Design review of the part built by this model. Coordinates are the model's own, in mm. A direction names the side the tool comes from. Coordinates: 2 decimals unless noted, no trailing zeros. Order: outer loops, then holes, each group sorted by start corner. A loop starts at its lowest first (then second) coordinate and runs counter-clockwise, first axis right, second up. Notation, with made-up numbers: M -3.5,52 L 50.5,52 A20 ccw 50.5,78 Z; hole C 28,-39 d9. An arc over 180 degrees is marked long. Use CSV: the item, a comma, the result in double quotes.
```python
from build123d import *

# Parameters (mm, degrees)
CROQUIS1_W                = 209.55
CROQUIS1_H                = 146.05
SALIENTE_EXTRUIR1_DEPTH   = 3.1242
CROQUIS2_R                = 1.3335
CORTAR_EXTRUIR1_DEPTH     = 128.750584639
CROQUIS9_R                = 1.27
CORTAR_EXTRUIR6_DEPTH     = 128.750584639
CORTAR_EXTRUIR2_DEPTH     = 128.750584639
CROQUIS5_R                = 1.651
DRIVER_DEPTH              = 128.750584639
CROQUIS6_R                = 1.651
RASPI_DEPTH               = 128.750584639
CROQUIS8_R                = 1.27
DIFERENCIAL_TRASERO_DEPTH = 128.750584639
CROQUIS7_R                = 1.5875
CROQUIS7_W                = 11.1125
CROQUIS7_H                = 2.9972
CORTAR_EXTRUIR7_DEPTH     = 128.750584639
CROQUIS10_R               = 1.651
CROQUIS10_W               = 22.606
CROQUIS10_H               = 11.9888
CORTAR_EXTRUIR10_DEPTH    = 128.750584639
CORTAR_EXTRUIR11_DEPTH    = 128.750584639


with BuildPart() as part:
    # Croquis1 → Saliente-Extruir1 (new body)
    with BuildSketch(Plane.XY):
        Rectangle(CROQUIS1_W, CROQUIS1_H)
    extrude(amount=SALIENTE_EXTRUIR1_DEPTH)

    # Croquis2 → Cortar-Extruir1 (cut, through all)
    with BuildSketch(Plane.XY.offset(3.1242)):
        with BuildLine():
            ThreePointArc((80.5799125, 60.7314), (79.928852882, 61.877042778), (78.6114125, 61.904002767))
            Line((78.6114125, 61.904002767), (78.6114125, 59.558797233))
            ThreePointArc((78.6114125, 59.558797233), (79.928852882, 59.585757222), (80.5799125, 60.7314))
        make_face()
        with BuildLine():
            Line((78.6114125, 59.558797233), (78.6114125, 61.904002767))
            ThreePointArc((78.6114125, 61.904002767), (77.9129125, 60.7314), (78.6114125, 59.558797233))
        make_face()
        with Locations(Location((79.2464125, -60.7314, 0), (0, 0, 180))):
            Circle(CROQUIS2_R)
    extrude(amount=-CORTAR_EXTRUIR1_DEPTH, mode=Mode.SUBTRACT)

    # Croquis9 → Cortar-Extruir6 (cut, through all)
    with BuildSketch(Plane.XY.offset(3.1242)):
        with Locations((63.3206125, 37.6809)):
            Circle(CROQUIS9_R)
        with Locations((95.1722125, 37.6809)):
            Circle(CROQUIS9_R)
        with Locations(Location((95.1722125, -37.6809, 0), (0, 0, 180))):
            Circle(CROQUIS9_R)
        with Locations(Location((63.3206125, -37.6809, 0), (0, 0, 180))):
            Circle(CROQUIS9_R)
    extrude(amount=-CORTAR_EXTRUIR6_DEPTH, mode=Mode.SUBTRACT)

    # Croquis3 → Cortar-Extruir2 (cut, through all)
    with BuildSketch(Plane.XY.offset(3.1242)):
        with BuildLine():
            Line((38.1, 67.507041999), (38.1, 73.025))
            Line((38.1, 73.025), (31.75, 73.025))
            ThreePointArc((31.75, 73.025), (35.663372801, 71.675801268), (37.913779422, 68.201539629))
            ThreePointArc((37.913779422, 68.201539629), (38.003556568, 67.853397075), (38.1, 67.507041999))
        make_face()
        with BuildLine():
            Line((74.0870375, 73.025), (38.1, 73.025))
            Line((38.1, 73.025), (38.1, 67.507041999))
            ThreePointArc((38.1, 67.507041999), (44.836488972, 57.735545708), (56.09351875, 53.975))
            ThreePointArc((56.09351875, 53.975), (63.258442282, 54.43812298), (70.304123502, 55.81978439))
            ThreePointArc((70.304123502, 55.81978439), (73.03168636, 57.631625564), (74.0870375, 60.7314))
            Line((74.0870375, 60.7314), (74.0870375, 73.025))
        make_face()
        with BuildLine():
            Line((104.775, 73.025), (74.0870375, 73.025))
            Line((74.0870375, 73.025), (74.0870375, 60.7314))
            ThreePointArc((74.0870375, 60.7314), (77.605786537, 65.622974066), (83.362384549, 63.842336271))
            ThreePointArc((83.362384549, 63.842336271), (99.279214777, 33.668769191), (104.775, 5.82e-07))
            Line((104.775, 5.82e-07), (104.775, 73.025))
        make_face()
        with BuildLine():
            Line((104.775, -73.025), (104.775, 5.82e-07))
            ThreePointArc((104.775, 5.82e-07), (99.279214962, -33.668768639), (83.362384549, -63.842336271))
            ThreePointArc((83.362384549, -63.842336271), (77.605786537, -65.622974066), (74.0870375, -60.7314))
            Line((74.0870375, -60.7314), (74.0870375, -73.025))
            Line((74.0870375, -73.025), (104.775, -73.025))
        make_face()
        with BuildLine():
            Line((74.0870375, -73.025), (74.0870375, -60.7314))
            ThreePointArc((74.0870375, -60.7314), (73.03168636, -57.631625564), (70.304123502, -55.81978439))
            ThreePointArc((70.304123502, -55.81978439), (63.258442282, -54.43812298), (56.09351875, -53.975))
            ThreePointArc((56.09351875, -53.975), (44.836488972, -57.735545708), (38.1, -67.507041999))
            Line((38.1, -67.507041999), (38.1, -73.025))
            Line((38.1, -73.025), (74.0870375, -73.025))
        make_face()
        with BuildLine():
            ThreePointArc((37.913779422, -68.201539629), (35.663372801, -71.675801268), (31.75, -73.025))
            Line((31.75, -73.025), (38.1, -73.025))
            Line((38.1, -73.025), (38.1, -67.507041999))
            ThreePointArc((38.1, -67.507041999), (38.003556568, -67.853397075), (37.913779422, -68.201539629))
        make_face()
        with BuildLine():
            ThreePointArc((-104.775, 63.5), (-101.985192091, 70.235192091), (-95.25, 73.025))
            Line((-95.25, 73.025), (-104.775, 73.025))
            Line((-104.775, 73.025), (-104.775, 63.5))
        make_face()
        with BuildLine():
            Line((-104.775, -73.025), (-95.25, -73.025))
            ThreePointArc((-95.25, -73.025), (-101.985192091, -70.235192091), (-104.775, -63.5))
            Line((-104.775, -63.5), (-104.775, -73.025))
        make_face()
    extrude(amount=-CORTAR_EXTRUIR2_DEPTH, mode=Mode.SUBTRACT)

    # Croquis5 → Driver (cut, through all)
    with BuildSketch(Plane.XY.offset(3.1242)):
        with BuildLine():
            Line((12.47775, -19.2786), (-18.82775, -19.2786))
            ThreePointArc((-18.82775, -19.2786), (-19.389016008, -19.511083992), (-19.6215, -20.07235))
            Line((-19.6215, -20.07235), (-19.6215, -25.8826))
            ThreePointArc((-19.6215, -25.8826), (-20.55143597, -28.12766403), (-22.7965, -29.0576))
            Line((-22.7965, -29.0576), (-24.7015, -29.0576))
            ThreePointArc((-24.7015, -29.0576), (-28.293602448, -30.545497552), (-29.7815, -34.1376))
            Line((-29.7815, -34.1376), (-29.7815, -54.991))
            ThreePointArc((-29.7815, -54.991), (-28.293602448, -58.583102448), (-24.7015, -60.071))
            Line((-24.7015, -60.071), (-22.7965, -60.071))
            ThreePointArc((-22.7965, -60.071), (-20.55143597, -61.00093597), (-19.6215, -63.246))
            Line((-19.6215, -63.246), (-19.6215, -69.05625))
            ThreePointArc((-19.6215, -69.05625), (-19.389016008, -69.617516008), (-18.82775, -69.85))
            Line((-18.82775, -69.85), (12.47775, -69.85))
            ThreePointArc((12.47775, -69.85), (13.039016008, -69.617516008), (13.2715, -69.05625))
            Line((13.2715, -69.05625), (13.2715, -59.563))
            ThreePointArc((13.2715, -59.563), (14.350225725, -56.958725725), (16.9545, -55.88))
            Line((16.9545, -55.88), (19.05, -55.88))
            ThreePointArc((19.05, -55.88), (20.172532015, -55.415032015), (20.6375, -54.2925))
            Line((20.6375, -54.2925), (20.6375, -34.8361))
            ThreePointArc((20.6375, -34.8361), (20.172532015, -33.713567985), (19.05, -33.2486))
            Line((19.05, -33.2486), (16.9545, -33.2486))
            ThreePointArc((16.9545, -33.2486), (14.350225725, -32.169874275), (13.2715, -29.5656))
            Line((13.2715, -29.5656), (13.2715, -20.07235))
            ThreePointArc((13.2715, -20.07235), (13.039016008, -19.511083992), (12.47775, -19.2786))
        make_face()
        with Locations((17.0815, -24.7396)):
            Circle(CROQUIS5_R)
        with Locations((-23.0505, -24.6126)):
            Circle(CROQUIS5_R)
        with Locations(Location((17.0815, -64.389, 0), (0, 0, 180))):
            Circle(CROQUIS5_R)
        with Locations(Location((-23.0505, -64.516, 0), (0, 0, 180))):
            Circle(CROQUIS5_R)
    extrude(amount=-DRIVER_DEPTH, mode=Mode.SUBTRACT)

    # Croquis6 → RasPi (cut, through all)
    with BuildSketch(Plane.XY.offset(3.1242)):
        with Locations((-29.95, 48.8814)):
            Circle(CROQUIS6_R)
        with Locations((19.05, 48.8814)):
            Circle(CROQUIS6_R)
        with Locations((19.05, -9.1186)):
            Circle(CROQUIS6_R)
        with Locations((-29.95, -9.1186)):
            Circle(CROQUIS6_R)
    extrude(amount=-RASPI_DEPTH, mode=Mode.SUBTRACT)

    # Croquis8 → Diferencial trasero (cut, through all)
    with BuildSketch(Plane.XY.offset(3.1242)):
        with Locations((-93.98, 54.3306)):
            Circle(CROQUIS8_R)
        with Locations((-61.214, 28.0162)):
            Circle(CROQUIS8_R)
    extrude(amount=-DIFERENCIAL_TRASERO_DEPTH, mode=Mode.SUBTRACT)

    # Croquis7 → Cortar-Extruir7 (cut, through all)
    with BuildSketch(Plane.XY.offset(3.1242)):
        with Locations((-92.508859415, -52.4764)):
            Circle(CROQUIS7_R)
        with Locations((-71.871359415, -52.4764)):
            Circle(CROQUIS7_R)
        with Locations((-82.190109415, -52.4764)):
            Rectangle(CROQUIS7_W, CROQUIS7_H)
    extrude(amount=-CORTAR_EXTRUIR7_DEPTH, mode=Mode.SUBTRACT)

    # Croquis10 → Cortar-Extruir10 (cut, through all)
    with BuildSketch(Plane.XY.offset(3.1242)):
        with Locations((82.0674, 9.652)):
            Circle(CROQUIS10_R)
        with Locations((82.0674, 0)):
            Rectangle(CROQUIS10_W, CROQUIS10_H)
        with Locations((82.0674, -9.652)):
            Circle(CROQUIS10_R)
        Polygon((93.3704, -1.966579717), (93.3704, -2.54), (95.4024, -2.54), (95.4024, 2.54), (93.3704, 2.54), align=None)
    extrude(amount=-CORTAR_EXTRUIR10_DEPTH, mode=Mode.SUBTRACT)

    # Croquis11 → Cortar-Extruir11 (cut, through all)
    with BuildSketch(Plane.XY.offset(3.1242)):
        with BuildLine():
            Line((-61.62675, 63.8302), (-84.93125, 63.8302))
            ThreePointArc((-84.93125, 63.8302), (-85.492516008, 63.597716008), (-85.725, 63.03645))
            Line((-85.725, 63.03645), (-85.725, 52.0827))
            ThreePointArc((-85.725, 52.0827), (-85.957483992, 51.521433992), (-86.51875, 51.28895))
            Line((-86.51875, 51.28895), (-95.72625, 51.28895))
            ThreePointArc((-95.72625, 51.28895), (-96.287516008, 51.056466008), (-96.52, 50.4952))
            Line((-96.52, 50.4952), (-96.52, 30.7467))
            ThreePointArc((-96.52, 30.7467), (-96.287516008, 30.185433992), (-95.72625, 29.95295))
            Line((-95.72625, 29.95295), (-61.62675, 29.95295))
            ThreePointArc((-61.62675, 29.95295), (-61.065483992, 30.185433992), (-60.833, 30.7467))
            Line((-60.833, 30.7467), (-60.833, 63.03645))
            ThreePointArc((-60.833, 63.03645), (-61.065483992, 63.597716008), (-61.62675, 63.8302))
        make_face()
        with BuildLine():
            ThreePointArc((-95.25, 73.025), (-98.445006556, 72.473157644), (-101.2698, 70.881573881))
            ThreePointArc((-101.2698, 70.881573881), (-99.585538364, 71.085343471), (-98.679, 69.651311567))
            Line((-98.679, 69.651311567), (-98.679, 67.0052))
            ThreePointArc((-98.679, 67.0052), (-98.214032015, 65.882667985), (-97.0915, 65.4177))
            Line((-97.0915, 65.4177), (-49.4665, 65.4177))
            ThreePointArc((-49.4665, 65.4177), (-48.343967985, 65.882667985), (-47.879, 67.0052))
            Line((-47.879, 67.0052), (-47.879, 71.4375))
            ThreePointArc((-47.879, 71.4375), (-47.414032015, 72.560032015), (-46.2915, 73.025))
            Line((-46.2915, 73.025), (-95.25, 73.025))
        make_face()
        with BuildLine():
            ThreePointArc((-98.679, -69.651311567), (-99.585538364, -71.085343471), (-101.2698, -70.881573881))
            ThreePointArc((-101.2698, -70.881573881), (-98.445006556, -72.473157644), (-95.25, -73.025))
            Line((-95.25, -73.025), (-46.2915, -73.025))
            ThreePointArc((-46.2915, -73.025), (-47.414032015, -72.560032015), (-47.879, -71.4375))
            Line((-47.879, -71.4375), (-47.879, -67.0052))
            ThreePointArc((-47.879, -67.0052), (-48.343967985, -65.882667985), (-49.4665, -65.4177))
            Line((-49.4665, -65.4177), (-97.0915, -65.4177))
            ThreePointArc((-97.0915, -65.4177), (-98.214032015, -65.882667985), (-98.679, -67.0052))
            Line((-98.679, -67.0052), (-98.679, -69.651311567))
        make_face()
    extrude(amount=-CORTAR_EXTRUIR11_DEPTH, mode=Mode.SUBTRACT)


solid = part.part
```
(1) Add section B-B on z = 0.75. Give the number of separate pieces and of enclosed holes in the cut face, and give its area (3 significant figures).
The answers:
separate pieces,"1"
enclosed holes,"24"
area,"23,500 mm2"
(2) Clearance check with flat-ended pins moving along their axes: P1, Ø0.9, axis at x = -73, z = 1.5, coming from the -Y side; P2, Ø1.6, axis at x = 94, z = 1.5, coming from the +Y side; P3, Ø3, axis at x = 19.05, y = 48.88, coming from the -Z side; P4, Ø1, axis at x = 72, z = 1, coming from the +Y side. State where each tip first meets the part, or that it passes through.
The answers:
P1,"stops at y = -65.42"
P2,"stops at y = 48.14"
P3,"passes through"
P4,"stops at y = 57.04"
(3) For faces 4 (the face through (-28.254, -30.506, 1.584)), 5 (the face through (35.71, -71.64, 1.58)), list the 3-axis set-ups (+Z, -Z, +X, -X, +Y, -Y) from which the entire face can be reached by the end or side of a thin tool; tool diameter is ignored.
The answers:
face 4,"+Z, -Z"
face 5,"+Z, -Z, +X, -Y"
(4) Wall thickness on probe 1 along Y at (x, z) = (-84, 2.6) (3 decimals); probe 2 along Y at (x, z) = (19.05, 2.35) (3 decimals); probe 3 along Y at (x, z) = (-70.5, 0.9): over which ranges is each line inside the solid? List them lowest first.
The answers:
probe 1,"y = -65.418 to -53.975, -50.978 to 29.953, 63.83 to 65.418"
probe 2,"y = -73.025 to -55.88, -33.249 to -10.77, -7.468 to 47.23, 50.532 to 73.025"
probe 3,"y = -65.42 to -53.28, -51.68 to 29.95, 63.83 to 65.42"
(5) Add section A-A on y = 33. State the section outline as (x, z) points (3 decimals).
The answers:
outline,"M -104.775,0 L -96.52,0 L -96.52,3.124 L -104.775,3.124 Z; M -60.833,0 L 99.501,0 L 99.501,3.124 L -60.833,3.124 Z"
(6) The part is to be moulded in two halves that separate along Y. For faces 1 (the face through (-1, 1, 0)), 2 (the face through (-28.333, -58.543, 1.584)), 3 (the face through (77.521, 65.594, 1.584)), say which applies: pulls with the +Y half, pulls with the -Y half, needs draft (parallel to the pull), parting line crosses it, or undercut.
The answers:
face 1,"needs draft"
face 2,"undercut"
face 3,"pulls with the +Y half"
(7) Add section C-C on y = -45.5. State the section outline as (x, z) points (1 decimal).
The answers:
outline,"M -104.8,0 L -29.8,0 L -29.8,3.1 L -104.8,3.1 Z; M 20.6,0 L 94.5,0 L 94.5,3.1 L 20.6,3.1 Z"
